```python
from build123d import *

# Parameters (mm, degrees)
SKETCH1_R           = 3.55
SKETCH1_R_2         = 2.55
BOSS_EXTRUDE1_DEPTH = 3


with BuildPart() as part:
    # Sketch1 → Boss-Extrude1 (new body)
    with BuildSketch(Plane(origin=(0, 0, 0), x_dir=(1, 0, 0), z_dir=(0, 1, 0))):
        with BuildLine():
            Line((60.5, -44), (-60.5, -44))
            ThreePointArc((-60.5, -44), (-62.621320344, -43.121320344), (-63.5, -41))
            Line((-63.5, -41), (-63.5, 41))
            ThreePointArc((-63.5, 41), (-62.621320344, 43.121320344), (-60.5, 44))
            Line((-60.5, 44), (60.5, 44))
            ThreePointArc((60.5, 44), (62.621320344, 43.121320344), (63.5, 41))
            Line((63.5, 41), (63.5, -41))
            ThreePointArc((63.5, -41), (62.621320344, -43.121320344), (60.5, -44))
        make_face()
        with Locations((-39.85, 30.32)):
            Circle(SKETCH1_R, mode=Mode.SUBTRACT)
        with Locations((0, 10)):
            Circle(SKETCH1_R_2, mode=Mode.SUBTRACT)
        Circle(SKETCH1_R_2, mode=Mode.SUBTRACT)
        with Locations((10, 0)):
            Circle(SKETCH1_R_2, mode=Mode.SUBTRACT)
        with Locations((-10, 0)):
            Circle(SKETCH1_R_2, mode=Mode.SUBTRACT)
        with Locations((-49.85, 30.32)):
            Circle(SKETCH1_R, mode=Mode.SUBTRACT)
        with Locations((-49.85, 0)):
            Circle(SKETCH1_R, mode=Mode.SUBTRACT)
        with Locations((-49.85, -30.32)):
            Circle(SKETCH1_R, mode=Mode.SUBTRACT)
        with Locations((-20.32, 10)):
            Circle(SKETCH1_R_2, mode=Mode.SUBTRACT)
        with Locations((-30.32, 10)):
            Circle(SKETCH1_R_2, mode=Mode.SUBTRACT)
        with Locations((-14.825, 14.825)):
            Circle(SKETCH1_R_2, mode=Mode.SUBTRACT)
        with Locations((0, 20.32)):
            Circle(SKETCH1_R_2, mode=Mode.SUBTRACT)
        with Locations((-49.85, 20.32)):
            Circle(SKETCH1_R_2, mode=Mode.SUBTRACT)
        with Locations((-39.85, 20.32)):
            Circle(SKETCH1_R_2, mode=Mode.SUBTRACT)
        with Locations((-29.85, 20.32)):
            Circle(SKETCH1_R_2, mode=Mode.SUBTRACT)
        with Locations((-39.85, 0)):
            Circle(SKETCH1_R, mode=Mode.SUBTRACT)
        with Locations((14.825, 14.825)):
            Circle(SKETCH1_R_2, mode=Mode.SUBTRACT)
        with Locations((20.32, 10)):
            Circle(SKETCH1_R_2, mode=Mode.SUBTRACT)
        with Locations((30.32, 10)):
            Circle(SKETCH1_R_2, mode=Mode.SUBTRACT)
        with Locations((39.85, 30.32)):
            Circle(SKETCH1_R_2, mode=Mode.SUBTRACT)
        with Locations((49.85, 30.32)):
            Circle(SKETCH1_R_2, mode=Mode.SUBTRACT)
        with Locations((49.85, 0)):
            Circle(SKETCH1_R_2, mode=Mode.SUBTRACT)
        with Locations((30.32, -10)):
            Circle(SKETCH1_R_2, mode=Mode.SUBTRACT)
        with Locations((49.85, -30.32)):
            Circle(SKETCH1_R_2, mode=Mode.SUBTRACT)
        with Locations((29.85, 30.32)):
            Circle(SKETCH1_R_2, mode=Mode.SUBTRACT)
        with Locations((20.32, -10)):
            Circle(SKETCH1_R_2, mode=Mode.SUBTRACT)
        with Locations((0, -10)):
            Circle(SKETCH1_R_2, mode=Mode.SUBTRACT)
        with Locations((14.825, -14.825)):
            Circle(SKETCH1_R_2, mode=Mode.SUBTRACT)
        with Locations((-29.85, 0)):
            Circle(SKETCH1_R, mode=Mode.SUBTRACT)
        with Locations((-19.85, 20.32)):
            Circle(SKETCH1_R_2, mode=Mode.SUBTRACT)
        with Locations((-9.69, 20.32)):
            Circle(SKETCH1_R_2, mode=Mode.SUBTRACT)
        with Locations((9.69, 20.32)):
            Circle(SKETCH1_R_2, mode=Mode.SUBTRACT)
        with Locations((-19.85, 0)):
            Circle(SKETCH1_R, mode=Mode.SUBTRACT)
        with Locations((-14.825, -14.825)):
            Circle(SKETCH1_R_2, mode=Mode.SUBTRACT)
        with Locations((-20.32, -10)):
            Circle(SKETCH1_R_2, mode=Mode.SUBTRACT)
        with Locations((-30.32, -10)):
            Circle(SKETCH1_R_2, mode=Mode.SUBTRACT)
        with Locations((-29.85, 30.32)):
            Circle(SKETCH1_R, mode=Mode.SUBTRACT)
        with Locations((-19.85, 30.32)):
            Circle(SKETCH1_R, mode=Mode.SUBTRACT)
        with Locations((19.85, 30.32)):
            Circle(SKETCH1_R_2, mode=Mode.SUBTRACT)
        with Locations((19.85, 20.32)):
            Circle(SKETCH1_R_2, mode=Mode.SUBTRACT)
        with Locations((29.85, 20.32)):
            Circle(SKETCH1_R_2, mode=Mode.SUBTRACT)
        with Locations((39.85, 20.32)):
            Circle(SKETCH1_R_2, mode=Mode.SUBTRACT)
        with Locations((49.85, 20.32)):
            Circle(SKETCH1_R_2, mode=Mode.SUBTRACT)
        with Locations((39.85, 0)):
            Circle(SKETCH1_R_2, mode=Mode.SUBTRACT)
        with Locations((29.85, 0)):
            Circle(SKETCH1_R_2, mode=Mode.SUBTRACT)
        with Locations((19.85, 0)):
            Circle(SKETCH1_R_2, mode=Mode.SUBTRACT)
        with Locations((19.85, -30.32)):
            Circle(SKETCH1_R_2, mode=Mode.SUBTRACT)
        with Locations((29.85, -30.32)):
            Circle(SKETCH1_R_2, mode=Mode.SUBTRACT)
        with Locations((0, -20.32)):
            Circle(SKETCH1_R_2, mode=Mode.SUBTRACT)
        with Locations((39.85, -30.32)):
            Circle(SKETCH1_R_2, mode=Mode.SUBTRACT)
        with Locations((49.85, -20.32)):
            Circle(SKETCH1_R_2, mode=Mode.SUBTRACT)
        with Locations((39.85, -20.32)):
            Circle(SKETCH1_R_2, mode=Mode.SUBTRACT)
        with Locations((29.85, -20.32)):
            Circle(SKETCH1_R_2, mode=Mode.SUBTRACT)
        with Locations((19.85, -20.32)):
            Circle(SKETCH1_R_2, mode=Mode.SUBTRACT)
        with Locations((9.69, -20.32)):
            Circle(SKETCH1_R_2, mode=Mode.SUBTRACT)
        with Locations((-9.69, -20.32)):
            Circle(SKETCH1_R_2, mode=Mode.SUBTRACT)
        with Locations((-19.85, -20.32)):
            Circle(SKETCH1_R_2, mode=Mode.SUBTRACT)
        with Locations((-29.85, -20.32)):
            Circle(SKETCH1_R_2, mode=Mode.SUBTRACT)
        with Locations((-39.85, -20.32)):
            Circle(SKETCH1_R_2, mode=Mode.SUBTRACT)
        with Locations((-49.85, -20.32)):
            Circle(SKETCH1_R_2, mode=Mode.SUBTRACT)
        with Locations((-19.85, -30.32)):
            Circle(SKETCH1_R, mode=Mode.SUBTRACT)
        with Locations((-29.85, -30.32)):
            Circle(SKETCH1_R, mode=Mode.SUBTRACT)
        with Locations((-39.85, -30.32)):
            Circle(SKETCH1_R, mode=Mode.SUBTRACT)
        with BuildLine():
            Line((10, 27.82), (-10, 27.82))
            ThreePointArc((-10, 27.82), (-12.5, 30.32), (-10, 32.82))
            Line((-10, 32.82), (10, 32.82))
            ThreePointArc((10, 32.82), (12.5, 30.32), (10, 27.82))
        make_face(mode=Mode.SUBTRACT)
        with BuildLine():
            Line((3.25, 36.5), (-3.25, 36.5))
            ThreePointArc((-3.25, 36.5), (-4.75, 38), (-3.25, 39.5))
            Line((-3.25, 39.5), (3.25, 39.5))
            ThreePointArc((3.25, 39.5), (4.75, 38), (3.25, 36.5))
        make_face(mode=Mode.SUBTRACT)
        with BuildLine():
            Line((-16.75, 36.5), (-23.25, 36.5))
            ThreePointArc((-23.25, 36.5), (-24.75, 38), (-23.25, 39.5))
            Line((-23.25, 39.5), (-16.75, 39.5))
            ThreePointArc((-16.75, 39.5), (-15.25, 38), (-16.75, 36.5))
        make_face(mode=Mode.SUBTRACT)
        with BuildLine():
            Line((16.75, 36.5), (23.25, 36.5))
            ThreePointArc((23.25, 36.5), (24.75, 38), (23.25, 39.5))
            Line((23.25, 39.5), (16.75, 39.5))
            ThreePointArc((16.75, 39.5), (15.25, 38), (16.75, 36.5))
        make_face(mode=Mode.SUBTRACT)
        with BuildLine():
            Line((10, -27.82), (-10, -27.82))
            ThreePointArc((-10, -27.82), (-12.5, -30.32), (-10, -32.82))
            Line((-10, -32.82), (10, -32.82))
            ThreePointArc((10, -32.82), (12.5, -30.32), (10, -27.82))
        make_face(mode=Mode.SUBTRACT)
        with BuildLine():
            Line((-16.75, -36.5), (-23.25, -36.5))
            ThreePointArc((-23.25, -36.5), (-24.75, -38), (-23.25, -39.5))
            Line((-23.25, -39.5), (-16.75, -39.5))
            ThreePointArc((-16.75, -39.5), (-15.25, -38), (-16.75, -36.5))
        make_face(mode=Mode.SUBTRACT)
        with BuildLine():
            Line((3.25, -36.5), (-3.25, -36.5))
            ThreePointArc((-3.25, -36.5), (-4.75, -38), (-3.25, -39.5))
            Line((-3.25, -39.5), (3.25, -39.5))
            ThreePointArc((3.25, -39.5), (4.75, -38), (3.25, -36.5))
        make_face(mode=Mode.SUBTRACT)
        with BuildLine():
            Line((16.75, -36.5), (23.25, -36.5))
            ThreePointArc((23.25, -36.5), (24.75, -38), (23.25, -39.5))
            Line((23.25, -39.5), (16.75, -39.5))
            ThreePointArc((16.75, -39.5), (15.25, -38), (16.75, -36.5))
        make_face(mode=Mode.SUBTRACT)
    extrude(amount=BOSS_EXTRUDE1_DEPTH)


solid = part.part
```
Geometry: final body of the model. Coordinates: model frame, mm. A direction names the side the tool comes from. Coordinates: 2 decimals unless noted, no trailing zeros. Loops run counter-clockwise (first coordinate to the right, second up) from the corner with the lowest first, then second, coordinate; pieces in that order, holes last. Notation, with made-up numbers: M 61,-29.5 L 82,-29.5 A9 cw 82,-12.5 Z; hole C 22,-24 d10. An arc over 180 degrees is marked long. Put each result on its own line as item: value.
(1) First-contact query: pin 1 (3 mm diameter, centred on x = 0, z = 20.32, fed in from +Y). Flat tip, straight axial feed; report the tip coordinate or a pass-through.
Answer sheet:
pin 1: passes through
(2) Draft query along X for faces 3 (the face through (15.25, 1.48, 38.03)), 4 (the face through (-1, 1, -44)), 5 (the face through (-42.398, 1.479, 20.208)). Return one class per face: pulls with the +X half, pulls with the -X half, needs draft (parallel to the pull), parting line crosses it, or undercut.
Answer sheet:
face 3: undercut
face 4: needs draft
face 5: undercut
(3) Cut plane B-B on x = -39.85. Return the cut outline in (y, z), then the cut area to 4 significant figures.
Answer sheet:
outline: M 0,-44 L 3,-44 L 3,-33.87 L 0,-33.87 Z; M 0,-26.77 L 3,-26.77 L 3,-22.87 L 0,-22.87 Z; M 0,-17.77 L 3,-17.77 L 3,-3.55 L 0,-3.55 Z; M 0,3.55 L 3,3.55 L 3,17.77 L 0,17.77 Z; M 0,22.87 L 3,22.87 L 3,26.77 L 0,26.77 Z; M 0,33.87 L 3,33.87 L 3,44 L 0,44 Z
area: 169.5 mm^2
(4) Material intervals for probe 1 along Z at (x, y) = (49.85, 2.45); probe 2 along X at (y, z) = (2.5, 16); probe 3 along Z at (x, y) = (-24, 1.05), sorted ascending.
Answer sheet:
probe 1: z = -44 to -32.87, -27.77 to -22.87, -17.77 to -2.55, 2.55 to 17.77, 22.87 to 27.77, 32.87 to 44
probe 2: x = -63.5 to -17.09, -12.56 to 12.56, 17.09 to 63.5
probe 3: z = -44 to -39.3, -36.7 to 36.7, 39.3 to 44
(5) Access query for faces 1 (the face through (4.75, 1.48, -38.03)), 2 (the face through (1, 1, 44)). Directions: +Z, -Z, +X, -X, +Y, -Y. A direction counts if a zero-diameter tool reaches every point of the face in a straight line with its end or side. Return the directions, or none.
Answer sheet:
face 1: +Y, -Y
face 2: +Z, +X, -X, +Y, -Y
(6) Cut plane D-D on x = -20. State how many separate pieces and enclosed holes the cut face has, then the cut area to 3 significant figures.
Answer sheet:
separate pieces: 10
enclosed holes: 0
area: 121 mm^2
(7) Cut plane A-A on z = 38. Return the cut outline in (x, y), then the cut area to 4 significant figures.
Answer sheet:
outline: M -63.5,0 L -24.75,0 L -24.75,3 L -63.5,3 Z; M -15.25,0 L -4.75,0 L -4.75,3 L -15.25,3 Z; M 4.75,0 L 15.25,0 L 15.25,3 L 4.75,3 Z; M 24.75,0 L 63.5,0 L 63.5,3 L 24.75,3 Z
area: 295.5 mm^2
(8) Cut plane C-C on x = 49.85. Return the cut outline in (y, z), then the cut area to 4 significant figures.
Answer sheet:
outline: M 0,-44 L 3,-44 L 3,-32.87 L 0,-32.87 Z; M 0,-27.77 L 3,-27.77 L 3,-22.87 L 0,-22.87 Z; M 0,-17.77 L 3,-17.77 L 3,-2.55 L 0,-2.55 Z; M 0,2.55 L 3,2.55 L 3,17.77 L 0,17.77 Z; M 0,22.87 L 3,22.87 L 3,27.77 L 0,27.77 Z; M 0,32.87 L 3,32.87 L 3,44 L 0,44 Z
area: 187.5 mm^2
